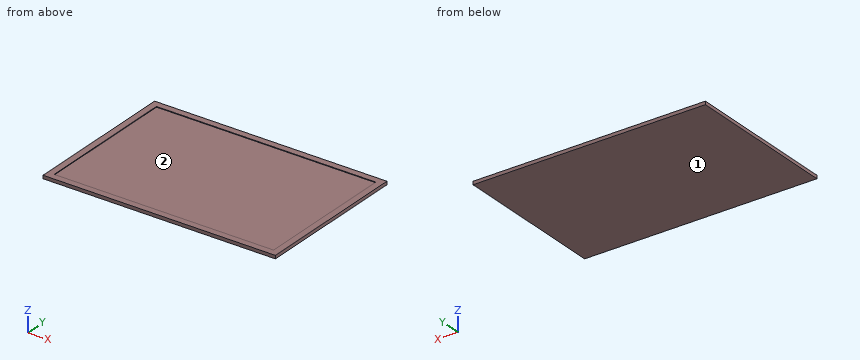
Autodesk Inventor part; units mm, degrees
ref_plane "YZ Plane" through (0, 0, 0) normal (1, 0, 0) x (0, 1, 0)
ref_plane "XZ Plane" through (0, 0, 0) normal (0, 1, 0) x (-1, 0, 0)
ref_plane "XY Plane" through (0, 0, 0) normal (0, 0, 1) x (1, 0, 0)
sketch "Sketch1" plane through (0, 0, 0) normal (0, 0, 1) x (1, 0, 0)
  line L0 (0, 0) -> (914.4, 0)
  line L1 (914.4, 0) -> (914.4, 609.6)
  line L2 (914.4, 609.6) -> (0, 609.6)
  line L3 (0, 609.6) -> (0, 0)
  dimension "d0" = 914.4
  dimension "d1" = 609.6
extrude "Extrusion1" add sketch "Sketch1" along normal blind 12.7
sketch "Sketch2" plane through (0, 0, 12.7) normal (0, 0, 1) x (1, 0, 0)
  line L0 (0, 609.6) -> (0, 0)
  line L1 (914.4, 609.6) -> (0, 609.6)
  line L2 (0, 0) -> (914.4, 0)
  line L3 (914.4, 0) -> (914.4, 609.6)
  line L4 (889, 25.4) -> (25.4, 25.4)
  line L5 (25.4, 25.4) -> (25.4, 584.2)
  line L6 (25.4, 584.2) -> (889, 584.2)
  line L7 (889, 584.2) -> (889, 25.4)
  dimension "d4" = 25.4
extrude "Extrusion2" cut sketch "Sketch2" against normal blind 2.54 contours L4 L5 L6 L7
properties part number "Ship area"
Source: CAD feature listing. Evaluate the final solid. Frame: model axes, mm. Face numbers are marked on the shaded views. Round coordinates to 2 decimals unless told otherwise and drop trailing zeros. Loops run counter-clockwise (first coordinate to the right, second up) from the corner with the lowest first, then second, coordinate; pieces in that order, holes last. Notation, with made-up numbers: (41.25, 50) - (55.25, 50) arc R20 ccw to (55.25, 88) - close; hole circle Ø1 at (60, 25.5). An arc over 180 degrees is marked (long way). Write item = value, one per line. Start each with the question number.
Item 1: Material intervals for line 1 (Y direction, x = 589, z = 12); line 2 (X direction, y = 33.5, z = 12); line 3 (Z direction, x = 362.5, y = 433), sorted ascending.
Item 2: Section query B-B on y = 40. Output: boundary loops of the cut face in (x, z), plus the area to 3 significant figures.
Item 3: Section query A-A on x = 590. Output: boundary loops of the cut face in (y, z).
Item 4: Mould query, pull axis Y, two halves, no side actions, for the marked faces 1 and 2. Classes: released by +Y, released by -Y, zero draft, split by the parting line, or undercut.
Item 5: First-contact query: pin 1 Ø10 at (x, y) = (225.5, 221.5) entering from +Z. Flat tip, straight axial feed; report the tip coordinate or a pass-through.
Results list:
q1.line_1 = 0 to 25.4, 584.2 to 609.6
q1.line_2 = 0 to 25.4, 889 to 914.4
q1.line_3 = 0 to 10.16
q2.outline = (0, 0) - (914.4, 0) - (914.4, 12.7) - (889, 12.7) - (889, 10.16) - (25.4, 10.16) - (25.4, 12.7) - (0, 12.7) - close
q2.area = 9,420 mm²
q3.outline = (0, 0) - (609.6, 0) - (609.6, 12.7) - (584.2, 12.7) - (584.2, 10.16) - (25.4, 10.16) - (25.4, 12.7) - (0, 12.7) - close
q4.face_1 = zero draft
q4.face_2 = undercut
q5.pin_1 = 10.16
